CAD build for the part. Positions are in the model's coordinates, mm. A direction names the side the tool comes from. Give positions to 0.01 mm unless a question says otherwise; leave off trailing zeros. Write each loop counter-clockwise with the first axis right and the second up, starting at its lowest first coordinate (ties: lowest second). Pieces come first, ordered by that corner, then holes. Notation, with made-up numbers: (13, -20.5) -> (38, -20.5) arc R12 ccw to (38, -12.5) -> close; hole circle Ø8 at (5, 3.5). An arc over 180 degrees is marked (long way). Answer as a JSON object with one key per item and string values.
Autodesk Fusion 360 part; units mm, degrees
sketch "outline" plane through (0, 0, 0) normal (0, 1, 0) x (1, 0, 0)
  line L0 (25, -60) -> (25, -40)
  arc A0 (25, -40) -> (15, -30) centre (15, -40) ccw
  line L1 (15, -30) -> (15, -10)
  line L2 (15, -10) -> (30, 0)
  line L3 (30, 0) -> (10, 0)
  line L4 (22, -60) -> (22, -40)
  arc A1 (22, -40) -> (12, -33.6754) centre (15, -40) ccw
  line L5 (12, -33.6754) -> (12, -8.3944)
  line L6 (12, -8.3944) -> (20.0917, -3)
  line L7 (20.0917, -3) -> (10, -3)
  line L8 (22, -60) -> (25, -60)
  line L9 (10, -3) -> (10, 0)
  line L10 (0, -60) -> (0, 0) construction
  dimension "d1" = -3
  dimension "d2" = 20
  dimension "d3" = 10
  dimension "d4" = 20
  dimension "d5" = 18.0278
  dimension "d6" = 20
revolve "Revolve1" add sketch "outline" angle 360 about axis through (0, 0, 60) along (0, 0, -1)
sketch "Sketch2" plane through (0, 0, 0) normal (0, 0, 1) x (1, 0, 0)
  circle A0 centre (0, 0) radius 10
extrude "Extrude1" add sketch "Sketch2" along normal blind 5
1) 3-axis set-ups, long thin cutter, end or side, ignore diameter. For faces 4 (the cylindrical face through (-2.17, 9.76, 3.99)), 5 (the flat face through (0, 0, 0)), 6 (the flat face through (-5, -9, 3)): which of +Z, -Z, +X, -X, +Y, -Y reach the whole face in a straight line?
Model answer:
{"face 4": "+Z", "face 5": "-Z, +X, -X, +Y, -Y", "face 6": "none"}
2) Mould opens along X. For faces 1 (the cylindrical face through (-4.769, 21.477, 49.86)), 2 (the flat face through (1.7, 22.1, 60)), 3 (the cylindrical face through (-14.985, -0.66, 19.86)) say: released by +X, released by -X, zero draft, split by the parting line, or undercut.
Model answer:
{"face 1": "undercut", "face 2": "zero draft", "face 3": "split by the parting line"}
3) Slice it at D-D (x = -17.5). State how many separate pieces and enclosed holes the cut face has, then the cut area to 3 significant figures.
Model answer:
{"separate pieces": "2", "enclosed holes": "1", "area": "557 mm2"}
4) Pin check, flat tips, straight feed: pin 1 (10 mm diameter, centred on x = -2.5, y = 0, fed in from +Z); pin 2 (4 mm diameter, centred on x = 22.5, y = 16.5, fed in from -Z); pin 3 (12 mm diameter, centred on x = -3.5, z = 43, fed in from -Y); pin 4 (1 mm diameter, centred on y = -0.5, z = 52.5, fed in from -X). Stop position of each tip, or through.
Model answer:
{"pin 1": "stops at z = 5", "pin 2": "stops at z = 0", "pin 3": "stops at y = -25", "pin 4": "stops at x = -25"}
5) Slice it at A-A (x = 0). List the corners of the cut face in (y, z).
Model answer:
{"outline": "(-30, 0) -> (30, 0) -> (15, 10) -> (15, 30) arc R10 ccw to (25, 40) -> (25, 60) -> (22, 60) -> (22, 40) arc R7 cw to (12, 33.68) -> (12, 8.39) -> (20.09, 3) -> (10, 3) -> (10, 5) -> (-10, 5) -> (-10, 3) -> (-20.09, 3) -> (-12, 8.39) -> (-12, 33.68) arc R7 cw to (-22, 40) -> (-22, 60) -> (-25, 60) -> (-25, 40) arc R10 ccw to (-15, 30) -> (-15, 10) -> close"}
6) Wall check: probe 1 along Y at (x, z) = (0, 26); probe 2 along X at (y, z) = (0, 46); probe 3 along X at (y, z) = (0.5, 15). Give the ranges that are in metal, low to high.
Model answer:
{"probe 1": "y = -15 to -12, 12 to 15", "probe 2": "x = -25 to -22, 22 to 25", "probe 3": "x = -14.99 to -11.99, 11.99 to 14.99"}
7) Slice it at C-C (z = 11.5). List the corners of the cut face in (x, y).
Model answer:
{"outline": "circle Ø30 at (0, 0); hole circle Ø24 at (0, 0)"}
